```python
from build123d import *

# Parameters (mm, degrees)
SKETCH1_W                 = 89
SKETCH1_H                 = 40
BOSS_EXTRUDE1_DEPTH       = 22
SKETCH2_W                 = 17
SKETCH2_H                 = 37
CUT_EXTRUDE1_DEPTH        = 20
SKETCH3_W                 = 17
SKETCH3_H                 = 2
BOSS_EXTRUDE2_DEPTH       = 17
BOSS_EXTRUDE10_DEPTH      = 2
BOSS_EXTRUDE10_DEPTH_BACK = 2
SKETCH4_W                 = 17
SKETCH4_H                 = 19
SKETCH4_R                 = 1.5
SKETCH5_W                 = 17
SKETCH5_H                 = 2
BOSS_EXTRUDE11_DEPTH      = 17
BOSS_EXTRUDE13_DEPTH      = 2
BOSS_EXTRUDE13_DEPTH_BACK = 2
SKETCH6_W                 = 17
SKETCH6_H                 = 25
SKETCH6_R                 = 1.5
SKETCH7_W                 = 0.1
SKETCH7_H                 = 2
CUT_EXTRUDE2_DEPTH        = 17
SKETCH8_W                 = 0.1
SKETCH8_H                 = 2
CUT_EXTRUDE11_DEPTH       = 17
SKETCH10_W                = 17
SKETCH10_H                = 5
SKETCH10_H_2              = 6
BOSS_EXTRUDE14_DEPTH      = 5
SKETCH11_W                = 0.1
SKETCH11_H                = 20
CUT_EXTRUDE12_DEPTH       = 17
SKETCH12_W                = 17
SKETCH12_H                = 5
BOSS_EXTRUDE15_DEPTH      = 5
SKETCH13_W                = 0.1
SKETCH13_H                = 26
CUT_EXTRUDE13_DEPTH       = 17


with BuildPart() as part:
    # Sketch1 → Boss-Extrude1 (new body)
    with BuildSketch(Plane.XY):
        Rectangle(SKETCH1_W, SKETCH1_H)
    extrude(amount=BOSS_EXTRUDE1_DEPTH)

    # Sketch2 → Cut-Extrude1 (cut)
    with BuildSketch(Plane.XY.offset(22)):
        with Locations((-36, 0)):
            Rectangle(SKETCH2_W, SKETCH2_H)
        with Locations((36, 0)):
            Rectangle(SKETCH2_W, SKETCH2_H)
    extrude(amount=-CUT_EXTRUDE1_DEPTH, mode=Mode.SUBTRACT)

    # Sketch3 → Boss-Extrude2 (add)
    with BuildSketch(Plane.XY.offset(2)):
        with Locations((-36, 9)):
            Rectangle(SKETCH3_W, SKETCH3_H)
        with Locations((-36, 2)):
            Rectangle(SKETCH3_W, SKETCH3_H)
        with Locations((-36, -6)):
            Rectangle(SKETCH3_W, SKETCH3_H)
        with Locations((-36, -13)):
            Rectangle(SKETCH3_W, SKETCH3_H)
    extrude(amount=BOSS_EXTRUDE2_DEPTH)

    # Sketch4 → Boss-Extrude10 (add, two sides: drawn at the far end of the back side and taken through both)
    with BuildSketch(Plane.XY.offset(19).offset(-BOSS_EXTRUDE10_DEPTH_BACK)):
        with Locations((-36, -2)):
            Rectangle(SKETCH4_W, SKETCH4_H)
        with Locations((-36, 5.5)):
            Circle(SKETCH4_R, mode=Mode.SUBTRACT)
        with Locations((-36, -2)):
            Circle(SKETCH4_R, mode=Mode.SUBTRACT)
        with Locations((-36, -9.5)):
            Circle(SKETCH4_R, mode=Mode.SUBTRACT)
    extrude(amount=BOSS_EXTRUDE10_DEPTH + BOSS_EXTRUDE10_DEPTH_BACK)

    # Sketch5 → Boss-Extrude11 (add)
    with BuildSketch(Plane.XY.offset(2)):
        with Locations((36, 16.778017119)):
            Rectangle(SKETCH5_W, SKETCH5_H)
        with Locations((36, 9.778017119)):
            Rectangle(SKETCH5_W, SKETCH5_H)
        with Locations((36, 2.778017119)):
            Rectangle(SKETCH5_W, SKETCH5_H)
        with Locations((36, -4.221982881)):
            Rectangle(SKETCH5_W, SKETCH5_H)
        with Locations((36, -11.221982881)):
            Rectangle(SKETCH5_W, SKETCH5_H)
    extrude(amount=BOSS_EXTRUDE11_DEPTH)

    # Sketch6 → Boss-Extrude13 (add, two sides: drawn at the far end of the back side and taken through both)
    with BuildSketch(Plane.XY.offset(19).offset(-BOSS_EXTRUDE13_DEPTH_BACK)):
        with Locations((36, 2.778017119)):
            Rectangle(SKETCH6_W, SKETCH6_H)
        with Locations((36, 13.278017119)):
            Circle(SKETCH6_R, mode=Mode.SUBTRACT)
        with Locations((36, 6.278017119)):
            Circle(SKETCH6_R, mode=Mode.SUBTRACT)
        with Locations((36, -0.721982881)):
            Circle(SKETCH6_R, mode=Mode.SUBTRACT)
        with Locations((36, -7.721982881)):
            Circle(SKETCH6_R, mode=Mode.SUBTRACT)
    extrude(amount=BOSS_EXTRUDE13_DEPTH + BOSS_EXTRUDE13_DEPTH_BACK)

    # Sketch7 → Cut-Extrude2 (cut)
    with BuildSketch(Plane.ZY.offset(44.5)):
        with Locations((2.05, 9)):
            Rectangle(SKETCH7_W, SKETCH7_H)
        with Locations((2.05, 2)):
            Rectangle(SKETCH7_W, SKETCH7_H)
        with Locations((2.05, -6)):
            Rectangle(SKETCH7_W, SKETCH7_H)
        with Locations((2.05, -13)):
            Rectangle(SKETCH7_W, SKETCH7_H)
        with Locations((16.95, -6)):
            Rectangle(SKETCH7_W, SKETCH7_H)
        with Locations((16.95, 2)):
            Rectangle(SKETCH7_W, SKETCH7_H)
    extrude(amount=-CUT_EXTRUDE2_DEPTH, mode=Mode.SUBTRACT)

    # Sketch8 → Cut-Extrude11 (cut)
    with BuildSketch(Plane(origin=(44.5, 0, 0), x_dir=(0, 0, -1), z_dir=(1, 0, 0))):
        with Locations((-2.05, -4.221982881)):
            Rectangle(SKETCH8_W, SKETCH8_H)
        with Locations((-16.95, -4.221982881)):
            Rectangle(SKETCH8_W, SKETCH8_H)
        with Locations((-16.95, 2.778017119)):
            Rectangle(SKETCH8_W, SKETCH8_H)
        with Locations((-16.95, 9.778017119)):
            Rectangle(SKETCH8_W, SKETCH8_H)
        with Locations((-2.05, 16.778017119)):
            Rectangle(SKETCH8_W, SKETCH8_H)
        with Locations((-2.05, 9.778017119)):
            Rectangle(SKETCH8_W, SKETCH8_H)
        with Locations((-2.05, 2.778017119)):
            Rectangle(SKETCH8_W, SKETCH8_H)
        with Locations((-2.05, -11.221982881)):
            Rectangle(SKETCH8_W, SKETCH8_H)
    extrude(amount=-CUT_EXTRUDE11_DEPTH, mode=Mode.SUBTRACT)

    # Sketch10 → Boss-Extrude14 (add)
    with BuildSketch(Plane.XY.offset(2)):
        with Locations((-36, 5.5)):
            Rectangle(SKETCH10_W, SKETCH10_H)
        with Locations((-36, -2)):
            Rectangle(SKETCH10_W, SKETCH10_H_2)
        with Locations((-36, -9.5)):
            Rectangle(SKETCH10_W, SKETCH10_H)
    extrude(amount=BOSS_EXTRUDE14_DEPTH)

    # Sketch11 → Cut-Extrude12 (cut)
    with BuildSketch(Plane.ZY.offset(44.5)):
        with Locations((2.05, -2)):
            Rectangle(SKETCH11_W, SKETCH11_H)
    extrude(amount=-CUT_EXTRUDE12_DEPTH, mode=Mode.SUBTRACT)

    # Sketch12 → Boss-Extrude15 (add)
    with BuildSketch(Plane.XY.offset(2)):
        with Locations((36, 13.278017119)):
            Rectangle(SKETCH12_W, SKETCH12_H)
        with Locations((36, 6.278017119)):
            Rectangle(SKETCH12_W, SKETCH12_H)
        with Locations((36, -0.721982881)):
            Rectangle(SKETCH12_W, SKETCH12_H)
        with Locations((36, -7.721982881)):
            Rectangle(SKETCH12_W, SKETCH12_H)
    extrude(amount=BOSS_EXTRUDE15_DEPTH)

    # Sketch13 → Cut-Extrude13 (cut)
    with BuildSketch(Plane(origin=(44.5, 0, 0), x_dir=(0, 0, -1), z_dir=(1, 0, 0))):
        with Locations((-2.05, 2.778017119)):
            Rectangle(SKETCH13_W, SKETCH13_H)
    extrude(amount=-CUT_EXTRUDE13_DEPTH, mode=Mode.SUBTRACT)


solid = part.part
```
The model under review builds one solid part; all positions refer to its coordinate system, in mm. A direction names the side the tool comes from. Round coordinates to 2 decimals unless told otherwise and drop trailing zeros. Loops run counter-clockwise (first coordinate to the right, second up) from the corner with the lowest first, then second, coordinate; pieces in that order, holes last. Notation, with made-up numbers: (73.25, 2) -> (86.25, 2) arc R14 ccw to (86.25, 12) -> close; hole circle Ø2 at (21.5, 4.25). An arc over 180 degrees is marked (long way). Answer as a JSON object with one key per item and string values. Group by question number.
1) We need section B-B on x = 36. Give the number of separate pieces and of enclosed holes in the cut face, then the cut area to 3 significant figures.
2) For pin 1 Ø1 at (x, y) = (-38.5, -5.5) entering from +Z; pin 2 Ø3 at (y, z) = (-8, 12.5) entering from +X; pin 3 Ø1.6 at (x, y) = (33, 17) entering from +Z, all flat-tipped, find the tip position at first contact; note any pin that passes through.
3) For line 1 (Y direction, x = -33, z = 14.75); line 2 (Y direction, x = -36, z = 19.55); line 3 (Z direction, x = -36.5, y = -18), list the stretches that pass through material, from the lowest coordinate up. Write a range as [from, to].
4) Mouldability with a two-part tool opening along Y and no side actions: class faces 1 (the face through (44.5, 3, 9)), 2 (the face through (-36, 3, 12)), 3 (the face through (-36, 8, 13)), 4 (the face through (-1, 20, 11)) as released by +Y, released by -Y, zero draft, split by the parting line, or undercut.
5) For faces 5 (the face through (36, 8.778, 12)), 6 (the face through (-44.5, -2, 19)), 7 (the face through (-34, -2, 17)), 8 (the face through (36, 17.778, 10)), 9 (the face through (-36, 9, 19)), list the 3-axis set-ups (+Z, -Z, +X, -X, +Y, -Y) from which the entire face can be reached by the end or side of a thin tool; tool diameter is ignored.
6) We need section A-A on x = -31. Write out the cut boundary in (y, z).
Result set:
{
 "1": {"separate pieces": "7", "enclosed holes": "0", "area": "446 mm²"},
 "2": {"pin 1": "z = 21", "pin 2": "x = 27.5", "pin 3": "z = 19"},
 "3": {"line 1": "[-20, -18.5], [-14, -12], [-7, -5], [1, 3], [8, 10], [18.5, 20]", "line 2": "[-20, -18.5], [-11.5, -11], [-8, -3.5], [-0.5, 4], [7, 7.5], [18.5, 20]", "line 3": "[0, 2]"},
 "4": {"face 1": "zero draft", "face 2": "undercut", "face 3": "undercut", "face 4": "released by +Y"},
 "5": {"face 5": "+X", "face 6": "+Z, -Z, -X, +Y, -Y", "face 7": "-X", "face 8": "+Z, +X", "face 9": "+Z, -X"},
 "6": {"outline": "(-20, 0) -> (20, 0) -> (20, 22) -> (18.5, 22) -> (18.5, 2) -> (-18.5, 2) -> (-18.5, 22) -> (-20, 22) -> close; (-14, 2.1) -> (10, 2.1) -> (10, 19) -> (8, 19) -> (8, 7) -> (3, 7) -> (3, 16.9) -> (1, 16.9) -> (1, 7) -> (-5, 7) -> (-5, 16.9) -> (-7, 16.9) -> (-7, 7) -> (-12, 7) -> (-12, 19) -> (-14, 19) -> close; (-11.5, 17) -> (7.5, 17) -> (7.5, 21) -> (-11.5, 21) -> close"}
}
